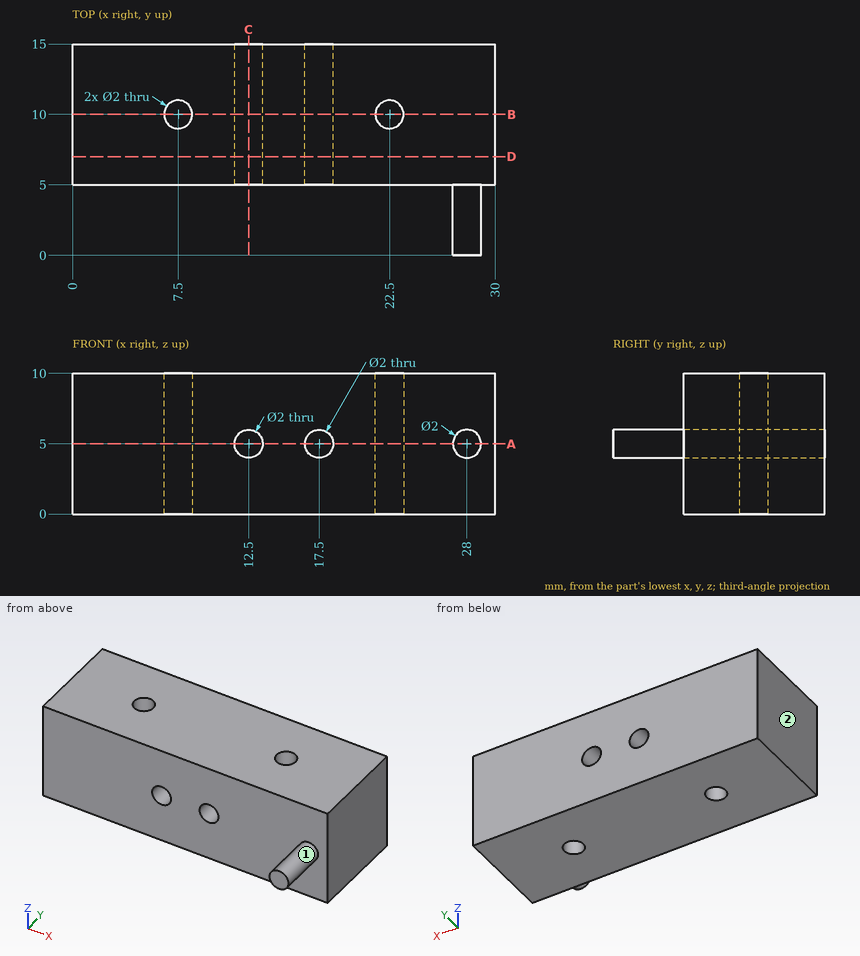
Job drawing, mm, ordinate dimensions from the low corner. One solid piece. A direction names the side the tool comes from. Coordinates: 2 decimals unless noted, no trailing zeros. Order: outer loops, then holes, each group sorted by start corner. A loop starts at its lowest first (then second) coordinate and runs counter-clockwise, first axis right, second up. Notation, with made-up numbers: M -36.75,42.5 L -28.75,42.5 A29 ccw -28.75,72.5 Z; hole C 61,-19.5 d4. An arc over 180 degrees is marked long. Return JSON: item names as keys, results as strings.
1. Saw through at B-B (y = 10). Give the cut face in (x, z).
Ans:
{"outline": "M 0,0 L 6.5,0 L 6.5,10 L 0,10 Z; M 8.5,0 L 21.5,0 L 21.5,10 L 8.5,10 Z; M 23.5,0 L 30,0 L 30,10 L 23.5,10 Z; hole C 12.5,5 d2; hole C 17.5,5 d2"}
2. Saw through at D-D (y = 7). Give the cut face in (x, z).
Ans:
{"outline": "M 0,0 L 30,0 L 30,10 L 0,10 Z; hole C 12.5,5 d2; hole C 17.5,5 d2"}
3. Saw through at A-A (z = 5). Give the cut face in (x, y), and give its area (3 significant figures).
Ans:
{"outline": "M 0,5 L 11.5,5 L 11.5,15 L 0,15 Z; M 13.5,5 L 16.5,5 L 16.5,15 L 13.5,15 Z; M 18.5,5 L 27,5 L 27,0 L 29,0 L 29,5 L 30,5 L 30,15 L 18.5,15 Z; hole C 7.5,10 d2; hole C 22.5,10 d2", "area": "264 mm^2"}
4. Drill centre lines: probe 1 along X at (y, z) = (7, 5.25); probe 2 along X at (y, z) = (9.5, 5); probe 3 along Y at (x, z) = (22.5, 2.25). Where is each one in solid material? Low to high.
Ans:
{"probe 1": "0 to 11.53, 13.47 to 16.53, 18.47 to 30", "probe 2": "0 to 6.63, 8.37 to 11.5, 13.5 to 16.5, 18.5 to 21.63, 23.37 to 30", "probe 3": "5 to 9, 11 to 15"}
5. Saw through at C-C (x = 12.5). Give the cut face in (y, z).
Ans:
{"outline": "M 5,0 L 15,0 L 15,4 L 5,4 Z; M 5,6 L 15,6 L 15,10 L 5,10 Z"}
6. Tool access for the marked faces 1 and 2: list every direction of +Z, -Z, +X, -X, +Y, -Y with a clear straight run to the whole face (end or side of a thin tool).
Ans:
{"face 1": "-Y", "face 2": "+Z, -Z, -X, +Y, -Y"}
